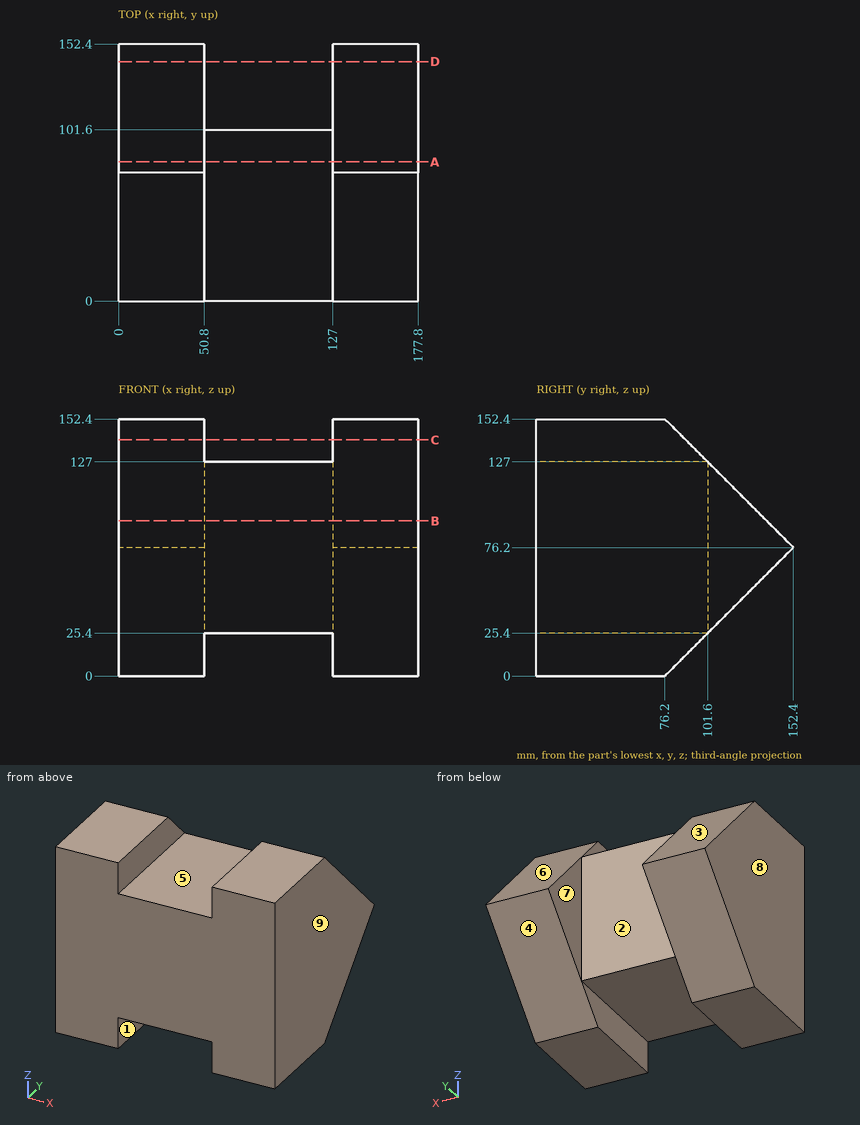
Verification items for this drawing (mm, ordinates from the low corner). A direction names the side the tool comes from. Give positions to 0.01 mm unless a question says otherwise; leave off trailing zeros. Write each loop counter-clockwise with the first axis right and the second up, starting at its lowest first coordinate (ties: lowest second). Pieces come first, ordered by that corner, then holes. Notation, with made-up numbers: (41, -22) -> (100, -22) arc R9 ccw to (100, -14) -> close; hole circle Ø11 at (-7.75, 40.25). An arc over 180 degrees is marked (long way). Use CSV: the item, a comma, the result in double quotes. Start each with the question number.
Q1. Tool access check on the marked faces 1, 2, 3, 4 and 5. Record the directions out of +Z, -Z, +X, -X, +Y, -Y that give a thin tool (end or side, any length) a straight path to the whole face; none if there is none.
Q2. Cross-section at B-B on z = 92. Enter the section's corners in (x, y).
Q3. Cross-section at D-D on y = 142. Enter the section's corners in (x, z).
Q4. Depth check by flat-ended pin: P1, Ø3, axis at x = 148.5, y = 126.5, coming from the +Z side; P2, Ø3, axis at x = 66.5, y = 21, coming from the -Z side; P3, Ø10, axis at x = 138.5, y = 129, coming from the +Z side. Enter the tip coordinate at first touch or a pass-through.
Q5. Release check for a two-part mould opening along X. For the marked faces 6, 7, 8 and 9 record: +X half, -X half, draft (parallel to the pull), parting line (faces both ways), or undercut.
Q6. Cross-section at A-A on y = 82.5. Enter the section's corners in (x, z).
Q7. Scan lines: line 1 along X through (y, z) = (132, 95.5); line 2 along Z through (x, y) = (87, 58); line 3 along Y through (x, z) = (124.5, 56.5). Record each from-to range of solid material in increasing order.
Q8. Cross-section at C-C on z = 140. Enter the section's corners in (x, y), and give its area (3 significant figures).
Working result:
1,face 1,"-Z, +Y, -Y"
1,face 2,"+Z, -Z, +Y"
1,face 3,"+Z, +X, -X, +Y"
1,face 4,"-Z, +X, -X, +Y"
1,face 5,"+Z, +Y, -Y"
2,outline,"(0, 0) -> (177.8, 0) -> (177.8, 136.6) -> (127, 136.6) -> (127, 101.6) -> (50.8, 101.6) -> (50.8, 136.6) -> (0, 136.6) -> close"
3,outline,"(0, 65.8) -> (50.8, 65.8) -> (50.8, 86.6) -> (0, 86.6) -> close; (127, 65.8) -> (177.8, 65.8) -> (177.8, 86.6) -> (127, 86.6) -> close"
4,P1,"stops at z = 103.6"
4,P2,"stops at z = 25.4"
4,P3,"stops at z = 104.6"
5,face 6,"draft"
5,face 7,"undercut"
5,face 8,"-X half"
5,face 9,"+X half"
6,outline,"(0, 6.3) -> (50.8, 6.3) -> (50.8, 25.4) -> (127, 25.4) -> (127, 6.3) -> (177.8, 6.3) -> (177.8, 146.1) -> (127, 146.1) -> (127, 127) -> (50.8, 127) -> (50.8, 146.1) -> (0, 146.1) -> close"
7,line 1,"x = 0 to 50.8, 127 to 177.8"
7,line 2,"z = 25.4 to 127"
7,line 3,"y = 0 to 101.6"
8,outline,"(0, 0) -> (50.8, 0) -> (50.8, 88.6) -> (0, 88.6) -> close; (127, 0) -> (177.8, 0) -> (177.8, 88.6) -> (127, 88.6) -> close"
8,area,"9,000 mm^2"
